Autodesk Inventor part; units mm, degrees
ref_plane "end1" through (-1037.7379, 0, 0) normal (1, 0, 0) x (0, 1, 0)
ref_plane "end2" through (1037.7379, 0, 0) normal (1, 0, 0) x (0, 1, 0)
ref_plane "XZ Plane" through (0, 0, 0) normal (0, 1, 0) x (-1, 0, 0)
sketch "Sketch1" plane through (0, 0, 0) normal (0, 0, 1) x (1, 0, 0)
  arc A0 (0, 890) -> (-1037.7379, 0) centre (0, -160) ccw
  arc A1 (1037.7379, 0) -> (0, 890) centre (0, -160) ccw
  arc A2 (0, 880) -> (-1027.6186, 0) centre (0, -160) ccw
  arc A3 (1027.6186, 0) -> (0, 880) centre (0, -160) ccw
  line L0 (1027.6186, 0) -> (1037.7379, 0)
  line L1 (-1037.7379, 0) -> (-1027.6186, 0)
  point P0 (0, 0)
  dimension "d0" = 0
  dimension "d1" = 0
  dimension "d2" = 0
  dimension "d3" = 160
  dimension "d6" = 890
  dimension "d8" = 1037.7379
  dimension "d10" = 0
  dimension "d11" = 10
  dimension "d12" = 0
revolve "Revolution2" add sketch "Sketch1" angle 90 about axis through (1027.6186, 0, 0) along (1, 0, 0)
ref_plane "end1" through (-1037.7379, 0, 0) normal (1, 0, 0) x (0, 1, 0)
sketch "Sketch3" plane through (-1037.7379, 0, 0) normal (1, 0, 0) x (0, 1, 0)
  line L0 (890, 0) -> (0, 0)
  line L1 (0, 890) -> (0, 0)
  line L2 (890, 0) -> (0, 0)
  line L3 (0, 0) -> (0, 890)
  line L4 (0, 890) -> (890, 890)
  line L5 (890, 890) -> (890, 0)
extrude "Extrusion1" cut sketch "Sketch3" along normal blind 1037.7379
ref_plane "end2" through (1037.7379, 0, 0) normal (1, 0, 0) x (0, 1, 0)
sketch "Sketch4" plane through (0, -160, 0) normal (0, 0, -1) x (-0.7590721, 0.6510065, 0)
  arc A0 (683.5569, 797.0257) -> (-683.5569, 797.0257) centre (0, 0) ccw
  arc A1 (677.0468, 789.435) -> (-675.8756, 790.438) centre (0, 0) ccw
  line L0 (677.0468, 789.435) -> (683.5569, 797.0257)
  line L1 (-675.8756, 790.438) -> (-683.5569, 797.0257)
  point P0 (104.161, 121.4515)
extrude "Extrusion2" add sketch "Sketch4" along normal blind 900
equation "\"d14\" = d8"
properties part number "cover2_sule_inner_extended"
The model under review builds one solid part; all positions refer to its coordinate system, in mm. A direction names the side the tool comes from. Coordinates: 2 decimals unless noted, no trailing zeros. Loops run counter-clockwise (first coordinate to the right, second up) from the corner with the lowest first, then second, coordinate; pieces in that order, holes last. Notation, with made-up numbers: (44.5, -12.75) -> (66.5, -12.75) arc R24 cw to (66.5, 23.25) -> close; hole circle Ø11 at (26, 30). An arc over 180 degrees is marked (long way). Use a Markdown table: item, result. Add a question column.
1. Add section A-A on z = -238. Write out the cut boundary in (x, y), plus the area to 3 significant figures.
2. To check wall thickness, follow line 1 (Y direction, x = 236, z = 511.5); line 2 (X direction, y = 735, z = -36); line 3 (Z direction, x = 914, y = 207.5). State the ranges of each line that lie inside material, in increasing order.
3. Clearance check with flat-ended pins moving along their axes: pin 1 Ø3 at (y, z) = (349.5, 146) entering from -X; pin 2 Ø2 at (y, z) = (169.5, 549.5) entering from +X; pin 3 Ø6 at (x, z) = (318.5, -17) entering from -Y. State where each tip first meets the part, or that it passes through.
4. Machinability: for faces 1 (the face through (684.26, 623.19, -443.7)), 2 (the face through (683, 632, -900)), which of the approach directions +Z, -Z, +X, -X, +Y, -Y give a long, thin tool a straight path to every point of the face, cutting with its end or side? Answer none if there is none.
Returned:
| question | item | result |
|---|---|---|
| 1 | outline | (0, 880) arc R1040 cw to (1027.62, 0) -> (1037.74, 0) arc R1050 ccw to (0, 890) -> close |
| 1 | area | 14,800 mm² |
| 2 | line 1 | y = 682.46 to 695.25 |
| 2 | line 2 | x = 529.69 to 549.07 |
| 2 | line 3 | z = 264.51 to 290.28 |
| 3 | pin 1 | stops at x = 888.66 |
| 3 | pin 2 | stops at x = 750.78 |
| 3 | pin 3 | stops at y = 829.06 |
| 4 | face 1 | -Z, -X, -Y |
| 4 | face 2 | -Z, +X, -X, +Y, -Y |
